Solid Edge part; units mm, degrees
sketch "Sketch1" plane through (0, 0, 0) normal (0, -1, 0) x (1, 0, 0)
  line L0 (10, 6) -> (-11, 6)
  line L1 (-11, 6) -> (-11, -6)
  line L2 (-11, -6) -> (10, -6)
  line L3 (10, -6) -> (10, 6)
  dimension "D1" = 10
  dimension "D2" = 11
extrude "Protrusion1" add sketch "Sketch1" along normal blind 1.5
sketch "Sketch2" plane through (0, -1.5, 0) normal (0, -1, 0) x (-1, 0, 0)
  line L0 (11, -6) -> (11, -4)
  line L1 (11, -4) -> (-10, -4)
  line L2 (-10, -4) -> (-10, -6)
  line L3 (-10, -6) -> (11, -6)
  line L4 (11, 6) -> (11, 4)
  line L5 (11, 4) -> (-10, 4)
  line L6 (-10, 4) -> (-10, 6)
  line L7 (-10, 6) -> (11, 6)
  dimension "D1" = 11
  dimension "D2" = 11
extrude "Extrusionsausprägung_7" add sketch "Sketch2" along normal blind 7
sketch "Sketch3" plane through (0, 0, 0) normal (0, 1, 0) x (1, 0, 0)
  arc A0 (-11, 4) -> (-11, -4) centre (-12.1667, 0) cw
  line L0 (-11, 4) -> (-11, -4)
  arc A1 (10, 4) -> (10, -4) centre (11.1667, 0) ccw
  line L1 (10, 4) -> (10, -4)
extrude "Cutout1" cut sketch "Sketch3" against normal through all
chamfer "Fase_4" distance 0.5 angle 45 2 edges at (-0.5, -8.5, 4) (-0.5, -8.5, -4)
properties material "ABS-Plastik, mittelfest"
Geometry check sheet. Reference: the model listing, model coordinates, mm. A direction names the side the tool comes from. Round coordinates to 2 decimals unless told otherwise and drop trailing zeros. Loops run counter-clockwise (first coordinate to the right, second up) from the corner with the lowest first, then second, coordinate; pieces in that order, holes last. Notation, with made-up numbers: (80.25, 58) -> (138.25, 58) arc R7 ccw to (138.25, 64) -> close; hole circle Ø8 at (46.25, -17.75). An arc over 180 degrees is marked (long way). Answer as a JSON object with one key per item and string values. Group by question number.
Item 1: Set-up check for faces 5 (the face through (10, -4, -5)), 6 (the face through (-1, -5, 4)): record each of +Z, -Z, +X, -X, +Y, -Y from which the full face is reachable in a straight line by a thin tool's end or side.
Item 2: Cross-section at D-D, the plane z = -3. Record the cut outline in (x, y).
Item 3: Cross-section at A-A, the plane y = -3. Record the cut outline in (x, z).
Item 4: Thickness scan on line 1 along Z through (x, y) = (-7, -7.75); line 2 along Y through (x, z) = (-7, 0.5); line 3 along Z through (x, y) = (8.25, -1). Record the ranges inside material, lowest first.
Item 5: Release check for a two-part mould opening along Z. For faces 1 (the face through (0, -4, 6)), 2 (the face through (0, 0, 0)), 3 (the face through (7, -1, 0)), 4 (the face through (-1, -4, -6)) record: pulls with the +Z half, pulls with the -Z half, needs draft (parallel to the pull), parting line crosses it, or undercut.
Item 6: Cross-section at B-B, the plane x = 4.5. Record the cut outline in (y, z), plus the area to 4 significant figures.
Item 7: Cross-section at C-C, the plane y = -1.25. Record the cut outline in (x, z), plus the area to 3 significant figures.
Item 8: Depth check by flat-ended pin: pin 1 Ø1.5 at (x, z) = (2.5, -3) entering from -Y. Enter the tip coordinate at first touch or a pass-through.
Determined:
{
 "1": {"face 5": "+Z, -Z, +X, +Y, -Y", "face 6": "+X, -X, -Y"},
 "2": {"outline": "(-9.28, -1.5) -> (8.28, -1.5) -> (8.28, 0) -> (-9.28, 0) -> close"},
 "3": {"outline": "(-11, -6) -> (10, -6) -> (10, -4) -> (-11, -4) -> close; (-11, 4) -> (10, 4) -> (10, 6) -> (-11, 6) -> close"},
 "4": {"line 1": "z = -6 to -4, 4 to 6", "line 2": "y = -1.5 to 0", "line 3": "z = -6 to -2.98, 2.98 to 6"},
 "5": {"face 1": "pulls with the +Z half", "face 2": "needs draft", "face 3": "undercut", "face 4": "pulls with the -Z half"},
 "6": {"outline": "(-8.5, -6) -> (0, -6) -> (0, 6) -> (-8.5, 6) -> (-8.5, 4.5) -> (-8, 4) -> (-1.5, 4) -> (-1.5, -4) -> (-8, -4) -> (-8.5, -4.5) -> close", "area": "45.75 mm²"},
 "7": {"outline": "(-11, -6) -> (10, -6) -> (10, -4) arc R4.17 cw to (10, 4) -> (10, 6) -> (-11, 6) -> (-11, 4) arc R4.17 cw to (-11, -4) -> close", "area": "217 mm²"},
 "8": {"pin 1": "stops at y = -1.5"}
}
